Here's how the part is built. I have some questions about the finished solid (model axes, mm). Face numbers are marked on the shaded views. A direction names the side the tool comes from. Round coordinates to 2 decimals unless told otherwise and drop trailing zeros. Loops run counter-clockwise (first coordinate to the right, second up) from the corner with the lowest first, then second, coordinate; pieces in that order, holes last. Notation, with made-up numbers: M 61,26.5 L 108,26.5 A12 cw 108,46.5 Z; hole C 83,32 d4. An arc over 180 degrees is marked long. Use a Markdown table: item, result.
```python
from build123d import *

# Parameters (mm, degrees)
F0_W      = 10
F0_H      = 30
F1_DEPTH  = 15
F2_W      = 30
F2_H      = 10
F3_DEPTH  = 40
F4_R      = 14.99999
F5_W      = 10
F5_H      = 30
F6_DEPTH  = 40
F7_R      = 14.99999
F8_R      = 10
F9_DEPTH  = 10
F10_R     = 10
F11_DEPTH = 10


# Not quite as in the source:
# - a fillet or chamfer is up to 0.001 mm smaller than in the source, because OpenCascade refuses the exact size


with BuildPart() as f1:
    # F0 (on Right) → F1 (new body, symmetric)
    with BuildSketch(Plane.YZ):
        Rectangle(F0_W, F0_H)
    extrude(amount=F1_DEPTH, both=True)

    # F2 (on face) → F3 (join)
    with BuildSketch(Plane.XZ.offset(5)):
        Rectangle(F2_W, F2_H)
    extrude(amount=F3_DEPTH)

    # F4 (radius 15 in the source; OpenCascade refuses exactly that, so slightly less here)
    f4_edges = [f1.edges().sort_by_distance(p)[0] for p in [
        (-15, -45, 0),
        (15, -45, 0),
    ]]
    fillet(f4_edges, radius=F4_R)

    # F5 (on face) → F6 (join)
    with BuildSketch(Plane(origin=(0, 5, 0), x_dir=(-1, 0, 0), z_dir=(0, 1, 0))):
        Rectangle(F5_W, F5_H)
    extrude(amount=F6_DEPTH)

    # F7 (radius 15 in the source; OpenCascade refuses exactly that, so slightly less here)
    f7_edges = [f1.edges().sort_by_distance(p)[0] for p in [
        (0, 45, 15),
        (0, 45, -15),
    ]]
    fillet(f7_edges, radius=F7_R)

    # F8 (on face) → F9 (cut, through all)
    with BuildSketch(Plane.XY.offset(5)):
        with Locations((0, -30)):
            Circle(F8_R)
    extrude(amount=-F9_DEPTH, mode=Mode.SUBTRACT)

    # F10 (on face) → F11 (cut, through all)
    with BuildSketch(Plane.YZ.offset(5)):
        with Locations((30, 0)):
            Circle(F10_R)
    extrude(amount=-F11_DEPTH, mode=Mode.SUBTRACT)


solid = f1.part
```
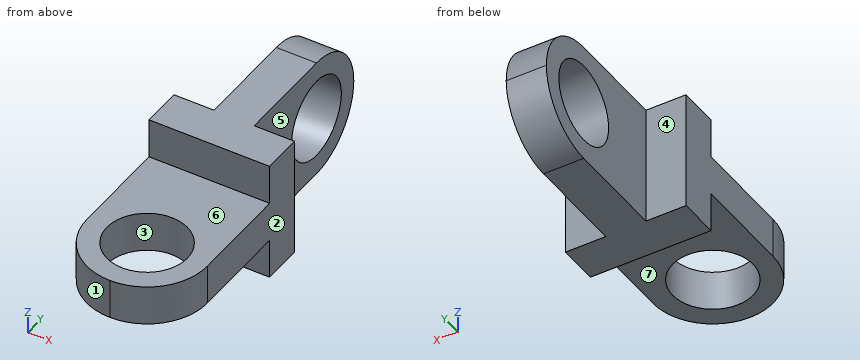
Q1. We'd pull the mould along Y, two halves only. Please class the marked faces 1, 2 and 3: pulls with the +Y half, pulls with the -Y half, needs draft (parallel to the pull), parting line crosses it, or undercut.
Return value:
| item | result |
|---|---|
| face 1 | pulls with the -Y half |
| face 2 | needs draft |
| face 3 | undercut |
Q2. Imagine slicing it at A-A, the plane x = 2.5. Give the number of separate pieces and of enclosed holes in the cut face, then the cut area to 3 significant figures.
Return value:
| item | result |
|---|---|
| separate pieces | 2 |
| enclosed holes | 1 |
| area | 1,290 mm^2 |
Q3. For the marked faces 4, 5, 6 and 7, which set-ups out of +Z, -Z, +X, -X, +Y, -Y let a thin tool reach every point of the face, with its end or its side?
Return value:
| item | result |
|---|---|
| face 4 | +Z, -Z, -X, +Y |
| face 5 | +Z, -Z, +X, +Y |
| face 6 | +Z, +X, -X, -Y |
| face 7 | -Z, +X, -X, -Y |
Q4. Imagine slicing it at D-D, the plane z = -12. Please give me the cut outline in (x, y), then the cut area to 3 significant figures.
Return value:
| item | result |
|---|---|
| outline | M -15,-5 L 15,-5 L 15,5 L 5,5 L 5,39 L -5,39 L -5,5 L -15,5 Z |
| area | 640 mm^2 |
Q5. Imagine slicing it at B-B, the plane z = 8.5. Please give me the cut outline in (x, y), then the cut area to 3 significant figures.
Return value:
| item | result |
|---|---|
| outline | M -15,-5 L 15,-5 L 15,5 L 5,5 L 5,24.73 L -5,24.73 L -5,5 L -15,5 Z; M -5,35.27 L 5,35.27 L 5,42.36 L -5,42.36 Z |
| area | 568 mm^2 |
Q6. I need wall thicknesses on line 1 (Y direction, x = -0.5, z = 0.5); line 2 (Y direction, x = 0, z = -1.75); line 3 (Z direction, x = -1.75, y = 30). Which ranges of each line are inside material? Lowest first, please. Write a range as from..to.
Return value:
| item | result |
|---|---|
| line 1 | y = -44.99..-39.99, -20.01..20.01, 39.99..44.99 |
| line 2 | y = -45..-40, -20..20.15, 39.85..44.9 |
| line 3 | z = -15..-10, 10..15 |
Q7. Imagine slicing it at C-C, the plane y = 21. Please give me the cut outline in (x, z).
Return value:
| item | result |
|---|---|
| outline | M -5,-15 L 5,-15 L 5,-4.36 L -5,-4.36 Z; M -5,4.36 L 5,4.36 L 5,15 L -5,15 Z |
Q8. Will these pins go through, and if not, where does the flat tip stop? P1, Ø15, axis at x = -5.5, y = -34.5, coming from the +Z side; P2, Ø8, axis at x = -3.5, z = 10.5, coming from the -Y side; P3, Ø3, axis at x = -11.5, z = -5.5, coming from the +Y side.
Return value:
| item | result |
|---|---|
| P1 | stops at z = 5 |
| P2 | stops at y = -5 |
| P3 | stops at y = 5 |
